```python
from build123d import *

# Parameters (mm, degrees)
F0_W     = 808.303834
F0_H     = 244.603918
F1_DEPTH = 201.93
F2_R     = 61.085102
F2_R_2   = 61.085249
F2_R_3   = 61.165723
F2_R_4   = 61.434425
F3_DEPTH = 45.72
F4_R     = 61.451385
F4_R_2   = 60.987438
F4_R_3   = 61.338193
F4_R_4   = 60.569848
F5_DEPTH = 45.72


with BuildPart() as f1:
    # F0 (on Front) → F1 (new body)
    with BuildSketch(Plane.XZ):
        Rectangle(F0_W, F0_H)
    extrude(amount=F1_DEPTH)

    # F2 (on face) → F3 (join)
    with BuildSketch(Plane.XY.offset(122.301959)):
        with Locations((-100.550018, -100.965)):
            Circle(F2_R)
        with Locations((100.115694, -100.965)):
            Circle(F2_R_2)
        with Locations((302.191652, -100.965)):
            Circle(F2_R_3)
        with Locations((-302.625977, -100.965)):
            Circle(F2_R_4)
    extrude(amount=F3_DEPTH)

    # F4 (on face) → F5 (cut)
    with BuildSketch(Plane(origin=(0, 0, -122.301959), x_dir=(1, 0, 0), z_dir=(0, 0, -1))):
        with Locations((303.214967, 100.965)):
            Circle(F4_R)
        with Locations((101.139009, 100.965)):
            Circle(F4_R_2)
        with Locations((-101.139016, 100.965)):
            Circle(F4_R_3)
        with Locations((-303.214975, 100.965)):
            Circle(F4_R_4)
    extrude(amount=-F5_DEPTH, mode=Mode.SUBTRACT)


solid = f1.part
```
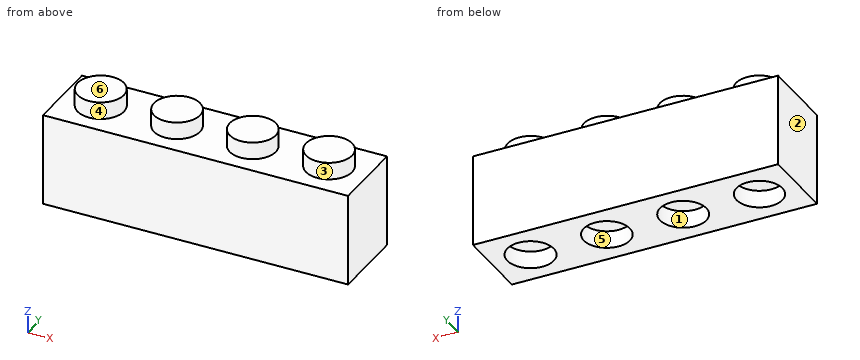
Source: CAD feature listing. Evaluate the final solid. Frame: model axes, mm. Face numbers are marked on the shaded views. A direction names the side the tool comes from. Round coordinates to 2 decimals unless told otherwise and drop trailing zeros. Loops run counter-clockwise (first coordinate to the right, second up) from the corner with the lowest first, then second, coordinate; pieces in that order, holes last. Notation, with made-up numbers: M 48,-33.5 L 73,-33.5 A24 cw 73,-7.5 Z; hole C 56.25,52.25 d10. An arc over 180 degrees is marked long. Use a Markdown table: item, result. Add a question column.
1. Section query B-B on y = -188.5. Return the cut outline in (x, z), then the cut area to 3 significant figures.
2. Section query A-A on x = -143. Return the cut outline in (y, z).
3. Section query D-D on x = 22.5. Return the cut outline in (y, z), then the cut area to 3 significant figures.
4. Reachability of the marked faces 1, 2 and 3 from +Z, -Z, +X, -X, +Y, -Y: full face, straight path, thin tool, end or side. Return the list, or none.
5. Line query: line 1 (Z direction, x = -140, y = -73.5); line 2 (X direction, y = -141, z = 129.5); line 3 (Z direction, x = 183, y = -155). Output: solid intervals per line, ascending.
6. Section query C-C on x = 110.5. Return the cut outline in (y, z).
7. Contact query for a flat-ended pin moving along its axis: P1, Ø8, axis at x = 169.5, y = -58, coming from the +Z side. Output: stop coordinate, or through.
8. Mould query, pull axis Y, two halves, no side actions, for the marked faces 4, 5 and 6. Classes: pulls with the +Y half, pulls with the -Y half, needs draft (parallel to the pull), parting line crosses it, or undercut.
Reported:
| question | item | result |
|---|---|---|
| 1 | outline | M -404.15,-122.3 L 404.15,-122.3 L 404.15,122.3 L -404.15,122.3 Z |
| 1 | area | 198,000 mm² |
| 2 | outline | M -201.93,-122.3 L -145.8,-122.3 L -145.8,-76.58 L -56.13,-76.58 L -56.13,-122.3 L 0,-122.3 L 0,122.3 L -57.04,122.3 L -57.04,168.02 L -144.89,168.02 L -144.89,122.3 L -201.93,122.3 Z |
| 3 | outline | M -201.93,-122.3 L 0,-122.3 L 0,122.3 L -201.93,122.3 Z |
| 3 | area | 49,400 mm² |
| 4 | face 1 | -Z |
| 4 | face 2 | +Z, -Z, -X, +Y, -Y |
| 4 | face 3 | +Z |
| 5 | line 1 | z = -76.58 to 168.02 |
| 5 | line 2 | x = -349.22 to -256.03, -146.69 to -54.41, 53.98 to 146.25, 255.95 to 348.43 |
| 5 | line 3 | z = -122.3 to 122.3 |
| 6 | outline | M -201.93,-122.3 L -161.23,-122.3 L -161.23,-76.58 L -40.7,-76.58 L -40.7,-122.3 L 0,-122.3 L 0,122.3 L -40.77,122.3 L -40.77,168.02 L -161.16,168.02 L -161.16,122.3 L -201.93,122.3 Z |
| 7 | P1 | stops at z = 122.3 |
| 8 | face 4 | parting line crosses it |
| 8 | face 5 | undercut |
| 8 | face 6 | needs draft |
